from build123d import *

# Parameters (mm, degrees)
SKETCH1_R           = 31.5
SKETCH1_R_2         = 22.625
BOSS_EXTRUDE1_DEPTH = 1.5
SKETCH2_R           = 1.4
BOSS_EXTRUDE2_DEPTH = 2.8


with BuildPart() as part:
    # Sketch1 → Boss-Extrude1 (new body)
    with BuildSketch(Plane(origin=(0, 0, 0), x_dir=(1, 0, 0), z_dir=(0, 1, 0))):
        with Locations(Location((0, 0, 0), (0, 0, 270))):
            Circle(SKETCH1_R)
        with Locations(Location((0, 0, 0), (0, 0, 270))):
            Circle(SKETCH1_R_2, mode=Mode.SUBTRACT)
    extrude(amount=BOSS_EXTRUDE1_DEPTH)

    # Sketch2 → Boss-Extrude2 (add)
    with BuildSketch(Plane(origin=(0, 0, 0), x_dir=(1, 0, 0), z_dir=(0, 1, 0))):
        with Locations(Location((-21.264622422, 16.637783303, 0), (0, 0, 270))):
            Circle(SKETCH2_R)
        with Locations(Location((9.252342519, 25.365215511, 0), (0, 0, 270))):
            Circle(SKETCH2_R)
        with Locations(Location((26.982884575, -0.961217985, 0), (0, 0, 270))):
            Circle(SKETCH2_R)
        with Locations(Location((7.423997262, -25.959280896, 0), (0, 0, 270))):
            Circle(SKETCH2_R)
        with Locations(Location((-22.394601934, -15.082499932, 0), (0, 0, 270))):
            Circle(SKETCH2_R)
    extrude(amount=-BOSS_EXTRUDE2_DEPTH)


solid = part.part
For this review, take the finished solid that the model builds, in its own axes (mm). A direction names the side the tool comes from. Give positions to 0.01 mm unless a question says otherwise; leave off trailing zeros. Write each loop counter-clockwise with the first axis right and the second up, starting at its lowest first coordinate (ties: lowest second). Pieces come first, ordered by that corner, then holes. Notation, with made-up numbers: (79, 21) -> (108, 21) arc R32 ccw to (108, 49) -> close; hole circle Ø8 at (47.5, 48). An arc over 180 degrees is marked (long way). Use CSV: the item, a comma, the result in double quotes.
Q1. To check wall thickness, follow probe 1 along X at (y, z) = (0.5, 0) (3 decimals); probe 2 along Y at (x, z) = (-22, 12.5); probe 3 along Z at (x, y) = (-9.5, 0.25). State the ranges of each line that lie inside material, in increasing order. Write a range as [from, to].
Conclusion:
probe 1,"[-31.5, -22.625], [22.625, 31.5]"
probe 2,"[0, 1.5]"
probe 3,"[-30.03, -20.53], [20.53, 30.03]"
Q2. Take a section at C-C, the plane y = -2.1. Write out the cut boundary in (x, z), then the cut area to 3 significant figures.
Conclusion:
outline,"circle Ø2.8 at (-22.39, 15.08); circle Ø2.8 at (-21.26, -16.64); circle Ø2.8 at (7.42, 25.96); circle Ø2.8 at (9.25, -25.37); circle Ø2.8 at (26.98, 0.96)"
area,"30.8 mm2"
Q3. Take a section at A-A, the plane x = 0. Write out the cut boundary in (y, z) (3 decimals).
Conclusion:
outline,"(0, -31.5) -> (1.5, -31.5) -> (1.5, -22.625) -> (0, -22.625) -> close; (0, 22.625) -> (1.5, 22.625) -> (1.5, 31.5) -> (0, 31.5) -> close"
Q4. For P1, Ø8, axis at x = -23, z = 21, coming from the -Y side, flat-tipped, find the tip position at first contact; note if it passes through.
Conclusion:
P1,"y = 0"
Q5. Take a section at B-B, the plane z = -20. Write out the cut boundary in (x, y).
Conclusion:
outline,"(-24.34, 0) -> (-10.58, 0) -> (-10.58, 1.5) -> (-24.34, 1.5) -> close; (10.58, 0) -> (24.34, 0) -> (24.34, 1.5) -> (10.58, 1.5) -> close"
Q6. Mouldability with a two-part tool opening along Z and no side actions: class faces 1 (the face through (27, -2.8, 1)), 2 (the face through (-21.974, -1.38, 16.418)), 3 (the face through (31.232, 0.74, -4.101)) as pulls with the +Z half, pulls with the -Z half, needs draft (parallel to the pull), parting line crosses it, or undercut.
Conclusion:
face 1,"needs draft"
face 2,"undercut"
face 3,"parting line crosses it"
Q7. Tool access review of faces 4 (the face through (25.616, -1.38, 0.658)), 5 (the face through (-22, -2.8, 15)): name each direction out of +Z, -Z, +X, -X, +Y, -Y from which nothing blocks a thin tool from reaching the whole face with its end or side.
Conclusion:
face 4,"-Y"
face 5,"+Z, -Z, +X, -X, -Y"
